Answer from the drawing. Dimensions are ordinates in mm from the lowest x, y and z of the part. A direction names the side the tool comes from. Coordinates: 2 decimals unless noted, no trailing zeros. Order: outer loops, then holes, each group sorted by start corner. A loop starts at its lowest first (then second) coordinate and runs counter-clockwise, first axis right, second up. Notation, with made-up numbers: (-8.5, 16) -> (50.5, 16) arc R28 ccw to (50.5, 35) -> close; hole circle Ø9 at (18, -13). An arc over 180 degrees is marked (long way). Use CSV: the item, a comma, the result in double quotes.
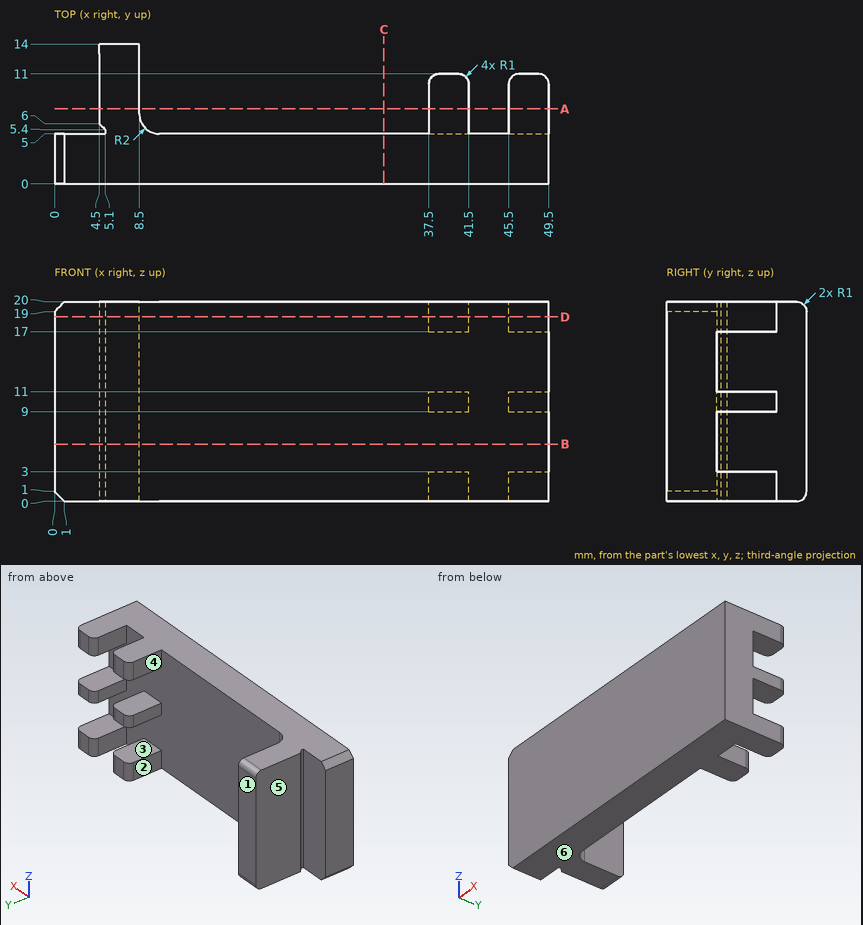
Item 1: A tool of negligible diameter and unlimited length cuts with its end or side. For the marked faces 1, 2 and 3, from which of +Z, -Z, +X, -X, +Y, -Y can it reach the whole face along a straight path? Write none if from no direction.
Return value:
face 1,"+Z, -Z, +X, -X, +Y"
face 2,"+Z, -Z, +Y"
face 3,"+X, +Y"
Item 2: Find section B-B, the plane z = 5.75. Give the vertices of the cut face in (x, y).
Return value:
outline,"(0, 0) -> (49.5, 0) -> (49.5, 5) -> (10.5, 5) arc R2 cw to (8.5, 7) -> (8.5, 14) -> (4.5, 14) -> (4.5, 6) -> (5.1, 5.4) -> (5.1, 5) -> (0, 5) -> close"
Item 3: Find section A-A, the plane y = 7.5. Give the vertices of the cut face in (x, z), then the cut area to 3 significant figures.
Return value:
outline,"(4.5, 0) -> (8.5, 0) -> (8.5, 20) -> (4.5, 20) -> close; (37.5, 0) -> (41.5, 0) -> (41.5, 3) -> (37.5, 3) -> close; (37.5, 9) -> (41.5, 9) -> (41.5, 11) -> (37.5, 11) -> close; (37.5, 17) -> (41.5, 17) -> (41.5, 20) -> (37.5, 20) -> close; (45.5, 0) -> (49.5, 0) -> (49.5, 3) -> (45.5, 3) -> close; (45.5, 9) -> (49.5, 9) -> (49.5, 11) -> (45.5, 11) -> close; (45.5, 17) -> (49.5, 17) -> (49.5, 20) -> (45.5, 20) -> close"
area,"144 mm^2"
Item 4: Find section C-C, the plane x = 33. Give the vertices of the cut face in (y, z), then the cut area to 3 significant figures.
Return value:
outline,"(0, 0) -> (5, 0) -> (5, 20) -> (0, 20) -> close"
area,"100 mm^2"
Item 5: Each of these flat-tipped pins is pushed along its axis until it touches: P1, Ø6, axis at y = 9.5, z = 16, coming from the -X side; P2, Ø2.5, axis at x = 2, z = 11.5, coming from the +Y side; P3, Ø2, axis at x = 47.5, z = 2, coming from the +Y side; P4, Ø2, axis at x = 10.5, y = 10.5, coming from the +Z side. Where does it stop, or does it pass through?
Return value:
P1,"stops at x = 4.5"
P2,"stops at y = 5"
P3,"stops at y = 11"
P4,"passes through"
Item 6: The mould has two halves that part along X. Classify the marked faces 4, 5 and 6: +X half, -X half, draft (parallel to the pull), parting line (faces both ways), or undercut.
Return value:
face 4,"undercut"
face 5,"-X half"
face 6,"draft"
Item 7: Straight lines are drawn through the part: line 1 along Y through (x, z) = (44, 8.5); line 2 along X through (y, z) = (9.75, 14.25); line 3 along X through (y, z) = (10.75, 2). For each, find the intervals that lie inside material, in ascending order.
Return value:
line 1,"y = 0 to 5"
line 2,"x = 4.5 to 8.5"
line 3,"x = 4.5 to 8.5, 37.84 to 41.16, 45.84 to 49.16"
Item 8: Find section D-D, the plane z = 18.5. Give the vertices of the cut face in (x, y).
Return value:
outline,"(0, 0) -> (49.5, 0) -> (49.5, 10) arc R1 ccw to (48.5, 11) -> (46.5, 11) arc R1 ccw to (45.5, 10) -> (45.5, 5) -> (41.5, 5) -> (41.5, 10) arc R1 ccw to (40.5, 11) -> (38.5, 11) arc R1 ccw to (37.5, 10) -> (37.5, 5) -> (10.5, 5) arc R2 cw to (8.5, 7) -> (8.5, 14) -> (4.5, 14) -> (4.5, 6) -> (5.1, 5.4) -> (5.1, 5) -> (0, 5) -> close"
